For this review, take the finished solid that the model builds, in its own axes (mm). A direction names the side the tool comes from. Round coordinates to 2 decimals unless told otherwise and drop trailing zeros. Write each loop counter-clockwise with the first axis right and the second up, starting at its lowest first coordinate (ties: lowest second). Pieces come first, ordered by that corner, then holes. Notation, with made-up numbers: (-25.5, 39) -> (-8.5, 39) arc R18 cw to (-8.5, 74) -> close; hole circle Ø11 at (-24, 46). An arc over 180 degrees is marked (long way). Write each question's results on one line, items separated by ' | '. Start each with the question number.
Item 1: Add section B-B (y = 4.25). State the section outline as (x, z) points, plus the area to 4 significant figures.
Item 2: Clearance check with flat-ended pins moving along their axes: pin 1 (5.5 mm diameter, centred on x = 12.34, z = 7.13, fed in from -Y); pin 2 (12 mm diameter, centred on x = 2.5, z = -17, fed in from -Y); pin 3 (2 mm diameter, centred on y = 7.5, z = -22.5, fed in from +X); pin 4 (2 mm diameter, centred on x = 3, y = 5.5, fed in from +Z). State where each tip first meets the part, or that it passes through.
Item 3: Add section A-A (z = 0). Count the separate pieces of the cut face and the enclosed holes in it, plus the area to 3 significant figures.
Item 4: To check wall thickness, follow line 1 along X through (y, z) = (8.5, -18); line 2 along Z through (x, y) = (10, 3.5); line 3 along Z through (x, y) = (10.5, 4.5). State the ranges of each line that lie inside material, in increasing order.
Item 5: The part is to be moulded in two halves that separate along X. For faces 3 (the flat face through (4, 11.5, -12)), 4 (the cylindrical face through (2.343, 10.996, 17.847)), 5 (the conical face through (15.17, 0.13, 8.96)), say which applies: +X half, -X half, draft (parallel to the pull), parting line (faces both ways), or undercut.
Item 6: Tool access review of faces 1 (the conical face through (-15.131, 8.377, 8.537)), 2 (the cylindrical face through (10.83, 9.98, 8.51)): name each direction out of +Z, -Z, +X, -X, +Y, -Y from which nothing blocks a thin tool from reaching the whole face with its end or side.
from build123d import *

# Parameters (mm, degrees)
CHAMFER_1_SIZE           = 0.25
SKETCH_2_R               = 2.1
SKETCH_2_R_2             = 2.05
CUT_EXTRUDE_1_DEPTH      = 4
SKETCH_3_R               = 6
CUT_EXTRUDE_2_DEPTH      = 9.5
PATTERN_CIRCULAR_1_COUNT = 3
SKETCH_4_R               = 2.1
CUT_EXTRUDE_3_DEPTH      = 12.5
PATTERN_CIRCULAR_2_COUNT = 6


with BuildPart() as part:
    # 草图1 → 旋转1 (revolve)
    with BuildSketch(Plane.XY):
        Polygon((-25, 0), (-17.5, 0), (-17.5, 8.5), (-11.5, 8.5), (-11.5, 11.5), (-18, 11.5), (-18, 10.5), (-28.5, 10.5), (-28.5, 8), (-25, 8), align=None)
    revolve(axis=Axis((0, 0, 0), (0, 1, 0)))

    # 倒角1
    chamfer_1_edges = [part.edges().sort_by_distance(p)[0] for p in [
        (11.5, 11.5, 0),
        (11.5, 8.5, 0),
        (17.5, 8.5, 0),
        (17.5, 0, 0),
        (25, 0, 0),
        (25, 8, 0),
        (28.5, 8, 0),
        (28.5, 10.5, 0),
        (18, 10.5, 0),
        (18, 11.5, 0),
    ]]
    chamfer(chamfer_1_edges, length=CHAMFER_1_SIZE)

    # 草图2 → 切除-拉伸1 (cut, through all)
    with BuildSketch(Plane.XZ.offset(-8.5)):
        with Locations((0, 15)):
            Circle(SKETCH_2_R)
        with Locations((0, -14.25)):
            Circle(SKETCH_2_R_2)
    cut_extrude_1 = extrude(amount=-CUT_EXTRUDE_1_DEPTH, mode=Mode.SUBTRACT)

    # 草图3 → 切除-拉伸2 (cut, through all)
    with BuildSketch(Plane.XZ.offset(-8.5)):
        with Locations((0, 15)):
            Circle(SKETCH_3_R)
    cut_extrude_2 = extrude(amount=CUT_EXTRUDE_2_DEPTH, mode=Mode.SUBTRACT)

    # 阵列(圆周)1: 切除-拉伸1, 切除-拉伸2 ×3 about axis
    pattern_circular_1_axis = Axis((0, 0, 0), (0, 1, 0))
    for i in range(1, PATTERN_CIRCULAR_1_COUNT):
        add(cut_extrude_1.rotate(pattern_circular_1_axis, i * 360 / PATTERN_CIRCULAR_1_COUNT), mode=Mode.SUBTRACT)
        add(cut_extrude_2.rotate(pattern_circular_1_axis, i * 360 / PATTERN_CIRCULAR_1_COUNT), mode=Mode.SUBTRACT)

    # 草图4 → 切除-拉伸3 (cut, through all)
    with BuildSketch(Plane.XZ):
        with Locations((10.5, 18.186533479)):
            Circle(SKETCH_4_R)
    cut_extrude_3 = extrude(amount=-CUT_EXTRUDE_3_DEPTH, mode=Mode.SUBTRACT)

    # 阵列(圆周)2: 切除-拉伸3 ×6 about axis
    pattern_circular_2_axis = Axis((0, 0, 0), (0, 1, 0))
    for i in range(1, PATTERN_CIRCULAR_2_COUNT):
        add(cut_extrude_3.rotate(pattern_circular_2_axis, i * 360 / PATTERN_CIRCULAR_2_COUNT), mode=Mode.SUBTRACT)


solid = part.part
Responses:
1) outline: circle Ø50 at (0, 0); hole circle Ø4.2 at (-21, 0); hole (-17.2, -3.22) arc R6 ccw to (-11.39, -13.28) arc R17.5 ccw to (11.39, -13.28) arc R6 ccw to (17.2, -3.22) arc R17.5 ccw to (5.81, 16.51) arc R6 ccw to (-5.81, 16.51) arc R17.5 ccw to start; hole circle Ø4.2 at (-10.5, -18.19); hole circle Ø4.2 at (-10.5, 18.19); hole circle Ø4.2 at (10.5, -18.19); hole circle Ø4.2 at (10.5, 18.19); hole circle Ø4.2 at (21, 0) | area: 825.5 mm^2
2) pin 1: stops at y = 8.5 | pin 2: stops at y = 0 | pin 3: stops at x = 18.31 | pin 4: stops at z = 24.92
3) separate pieces: 4 | enclosed holes: 0 | area: 124 mm^2
4) line 1: x = -22.1 to -12.59, -8.41 to 8.41, 12.59 to 22.1 | line 2: z = -22.91 to -20.23, -16.15 to -14.36, 14.36 to 16.15, 20.23 to 22.91 | line 3: z = -22.69 to -20.29, -16.09 to -14, 14 to 16.09, 20.29 to 22.69
5) face 3: draft | face 4: parting line | face 5: undercut
6) face 1: -Y | face 2: +Y, -Y
